Part model, mm, in its own coordinate system. Face numbers are marked on the shaded views. A direction names the side the tool comes from. Round coordinates to 2 decimals unless told otherwise and drop trailing zeros. Loops run counter-clockwise (first coordinate to the right, second up) from the corner with the lowest first, then second, coordinate; pieces in that order, holes last. Notation, with made-up numbers: (83.5, 50) - (139.5, 50) arc R14 ccw to (139.5, 56) - close; hole circle Ø8 at (84, 50). An arc over 180 degrees is marked (long way). Write each question's results on one line, items separated by ' | '. Start each with the question number.
(1) Cut at D-D, the plane y = 10. List the corners of the cut face in (x, z), then the cut area to 3 significant figures.
(2) Drill centre lines: L1, parallel to Y at x = 0, z = -4; L2, parallel to Y at x = 17, z = -16.5. Where is each one in solid material? Low to high.
(3) Tool access for the marked faces 1, 2, 3, 4 and 5: list every direction of +Z, -Z, +X, -X, +Y, -Y with a clear straight run to the whole face (end or side of a thin tool).
(4) Mould opens along Y. For the marked faces 6, 7, 8 and 9 say: released by +Y, released by -Y, zero draft, split by the parting line, or undercut.
(5) Cut at C-C, the plane y = 0. List the corners of the cut face in (x, z).
(6) Flat gauge pins, fed straight in: P1, Ø3, axis at x = 18.5, z = -30.5, coming from the -Y side; P2, Ø1, axis at x = 5, z = -30, coming from the +Y side; P3, Ø2.5, axis at y = 35, z = -2.5, coming from the +X side. Where does each tip first touch, or does it go through?
(7) Cut at B-B, the plane x = 15.5. List the corners of the cut face in (y, z), then the cut area to 3 significant figures.
(8) Cut at A-A, the plane z = -15. List the corners of the cut face in (x, y).
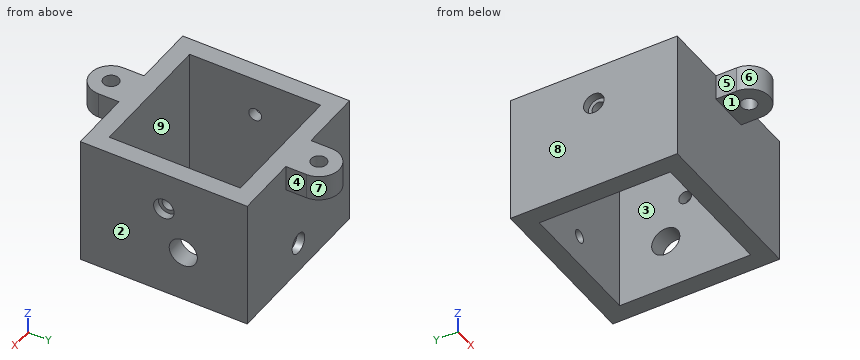
from build123d import *

# Parameters (mm, degrees)
ESBO_O1_W                = 51.2
ESBO_O1_H                = 51.2
RESSALTO_EXTRUS_O1_DEPTH = 50.6
ESBO_O1_3_R              = 3
RESSALTO_EXTRUS_O2_DEPTH = 10
ESBO_O3_R                = 5.5
CORTE_EXTRUS_O2_DEPTH    = 7
ESBO_O4_R                = 2.5
CORTE_EXTRUS_O3_DEPTH    = 96.77765919
ESBO_O5_R                = 4
CORTE_EXTRUS_O4_DEPTH    = 3
ESBO_O6_R                = 2.5
CORTE_EXTRUS_O5_DEPTH    = 7
ESBO_O7_R                = 4
CORTE_EXTRUS_O6_DEPTH    = 3


with BuildPart() as part:
    # Esboço1 → Ressalto-extrusão1 (new body)
    with BuildSketch(Plane.XY):
        Polygon((-8, 32.6), (-32.6, 32.6), (-32.6, -32.6), (-8, -32.6), (8, -32.6), (32.6, -32.6), (32.6, 32.6), (8, 32.6), align=None)
        Rectangle(ESBO_O1_W, ESBO_O1_H, mode=Mode.SUBTRACT)
    extrude(amount=-RESSALTO_EXTRUS_O1_DEPTH)

    # Esboço1<3> → Ressalto-extrusão2 (add)
    # profile 1 of 2: a face of its own
    with BuildSketch(Plane.XY):
        with BuildLine():
            Line((8, 32.6), (8, 40.6))
            ThreePointArc((8, 40.6), (0, 48.6), (-8, 40.6))
            Line((-8, 40.6), (-8, 32.6))
            Line((-8, 32.6), (8, 32.6))
        make_face()
        with Locations((0, 40.6)):
            Circle(ESBO_O1_3_R, mode=Mode.SUBTRACT)
    # profile 2 of 2: a face of its own
    with BuildSketch(Plane.XY):
        with BuildLine():
            ThreePointArc((8, -40.6), (0, -48.6), (-8, -40.6))
            Line((-8, -40.6), (-8, -32.6))
            Line((-8, -32.6), (8, -32.6))
            Line((8, -32.6), (8, -40.6))
        make_face()
        with Locations((0, -40.6)):
            Circle(ESBO_O1_3_R, mode=Mode.SUBTRACT)
    extrude(amount=-RESSALTO_EXTRUS_O2_DEPTH)

    # Esboço3 → Corte-extrusão2 (cut)
    with BuildSketch(Plane(origin=(32.6, 0, 0), x_dir=(0, 0, -1), z_dir=(1, 0, 0))):
        with Locations((30.6, 7.6)):
            Circle(ESBO_O3_R)
    extrude(amount=-CORTE_EXTRUS_O2_DEPTH, mode=Mode.SUBTRACT)

    # Esboço4 → Corte-extrusão3 (cut, through all)
    with BuildSketch(Plane(origin=(32.6, 0, 0), x_dir=(0, 0, -1), z_dir=(1, 0, 0))):
        with Locations((15, 0)):
            Circle(ESBO_O4_R)
    extrude(amount=-CORTE_EXTRUS_O3_DEPTH, mode=Mode.SUBTRACT)

    # Esboço5 → Corte-extrusão4 (cut)
    with BuildSketch(Plane(origin=(32.6, 0, 0), x_dir=(0, 0, -1), z_dir=(1, 0, 0))):
        with Locations((15, 0)):
            Circle(ESBO_O5_R)
    corte_extrus_o4 = extrude(amount=-CORTE_EXTRUS_O4_DEPTH, mode=Mode.SUBTRACT)

    # Espelhar1: Corte-extrusão4 across plane
    add(corte_extrus_o4.mirror(Plane(origin=(0, 0, 0), x_dir=(0, 0, 1), z_dir=(1, 0, 0))), mode=Mode.SUBTRACT)

    # Esboço6 → Corte-extrusão5 (cut)
    with BuildSketch(Plane(origin=(0, 32.6, 0), x_dir=(1, 0, 0), z_dir=(0, 1, 0))):
        with Locations(Location((0, 38.6, 0), (0, 0, 270))):
            Circle(ESBO_O6_R)
    extrude(amount=-CORTE_EXTRUS_O5_DEPTH, mode=Mode.SUBTRACT)

    # Esboço7 → Corte-extrusão6 (cut)
    with BuildSketch(Plane(origin=(0, 32.6, 0), x_dir=(1, 0, 0), z_dir=(0, 1, 0))):
        with Locations(Location((0, 38.6, 0), (0, 0, 270))):
            Circle(ESBO_O7_R)
    extrude(amount=-CORTE_EXTRUS_O6_DEPTH, mode=Mode.SUBTRACT)


solid = part.part
A:
1) outline: (-32.6, -50.6) - (-25.6, -50.6) - (-25.6, 0) - (-32.6, 0) - close; (25.6, -50.6) - (32.6, -50.6) - (32.6, -35.55) - (25.6, -35.55) - close; (25.6, -25.65) - (32.6, -25.65) - (32.6, 0) - (25.6, 0) - close | area: 639 mm2
2) L1: -48.6 to -43.6, -37.6 to -25.6, 25.6 to 37.6, 43.6 to 48.6 | L2: -32.6 to -25.6, 25.6 to 32.6
3) face 1: -Z, +X, -X, -Y | face 2: +Z, -Z, +X, +Y, -Y | face 3: +Z, -Z | face 4: +Z, -Z, +X, +Y | face 5: +Z, -Z, -X, -Y
4) face 6: released by -Y | face 7: released by +Y | face 8: zero draft | face 9: undercut
5) outline: (-32.6, -50.6) - (-25.6, -50.6) - (-25.6, -17.5) - (-29.6, -17.5) - (-29.6, -19) - (-32.6, -19) - close; (-32.6, -11) - (-29.6, -11) - (-29.6, -12.5) - (-25.6, -12.5) - (-25.6, 0) - (-32.6, 0) - close; (25.6, -50.6) - (32.6, -50.6) - (32.6, -19) - (29.6, -19) - (29.6, -17.5) - (25.6, -17.5) - close; (25.6, -12.5) - (29.6, -12.5) - (29.6, -11) - (32.6, -11) - (32.6, 0) - (25.6, 0) - close
6) P1: y = -32.6 | P2: y = 32.6 | P3: x = 8
7) outline: (-32.6, -50.6) - (-25.6, -50.6) - (-25.6, 0) - (-32.6, 0) - close; (25.6, -50.6) - (32.6, -50.6) - (32.6, 0) - (25.6, 0) - close | area: 708 mm2
8) outline: (-32.6, -32.6) - (32.6, -32.6) - (32.6, -4) - (29.6, -4) - (29.6, -2.5) - (25.6, -2.5) - (25.6, -25.6) - (-25.6, -25.6) - (-25.6, -2.5) - (-29.6, -2.5) - (-29.6, -4) - (-32.6, -4) - close; (-32.6, 4) - (-29.6, 4) - (-29.6, 2.5) - (-25.6, 2.5) - (-25.6, 25.6) - (25.6, 25.6) - (25.6, 2.5) - (29.6, 2.5) - (29.6, 4) - (32.6, 4) - (32.6, 32.6) - (-32.6, 32.6) - close
